Job drawing, mm, ordinate dimensions from the low corner. One solid piece. A direction names the side the tool comes from. Give positions to 0.01 mm unless a question says otherwise; leave off trailing zeros. Write each loop counter-clockwise with the first axis right and the second up, starting at its lowest first coordinate (ties: lowest second). Pieces come first, ordered by that corner, then holes. Notation, with made-up numbers: M 53.5,86 L 60.5,86 A37 ccw 60.5,124 Z; hole C 47.25,87.5 d8. An arc over 180 degrees is marked long. Answer as CSV lines item,"result". Start each with the question number.
Item 1: 3-axis set-ups, long thin cutter, end or side, ignore diameter. For the marked faces 5 and 6: which of +Z, -Z, +X, -X, +Y, -Y reach the whole face in a straight line?
Item 2: Wall check: L1, parallel to X at y = 33, z = 95.5 (3 decimals); L2, parallel to Z at x = 331, y = 35.5; L3, parallel to Z at x = 318, y = 17 (3 decimals). Give the ranges that are in metal, low to high. Write a range as from..to.
Item 3: Pin check, flat tips, straight feed: pin 1 (6 mm diameter, centred on x = 95.5, z = 20, fed in from -Y) (3 decimals); pin 2 (3 mm diameter, centred on x = 131.5, y = 14, fed in from -Z) (3 decimals). Stop position of each tip, or through.
Item 4: Band-saw the part on D-D, the plane y = 31. List the corners of the cut face in (x, z) (3 decimals), then the cut area to 3 significant figures.
Item 5: Band-saw the part on B-B, the plane z = 93. List the corners of the cut face in (x, y) (3 decimals).
Item 6: Band-saw the part on C-C, the plane z = 125. List the corners of the cut face in (x, y) (3 decimals).
Item 7: Band-saw the part on A-A, the plane x = 223. List the corners of the cut face in (y, z) (3 decimals), then the cut area to 3 significant figures.
Item 8: Two-plate mould, pull along X, no slides. Class the marked faces 1, 2, 3 and 4: +X half, -X half, draft (parallel to the pull), parting line (faces both ways), or undercut.
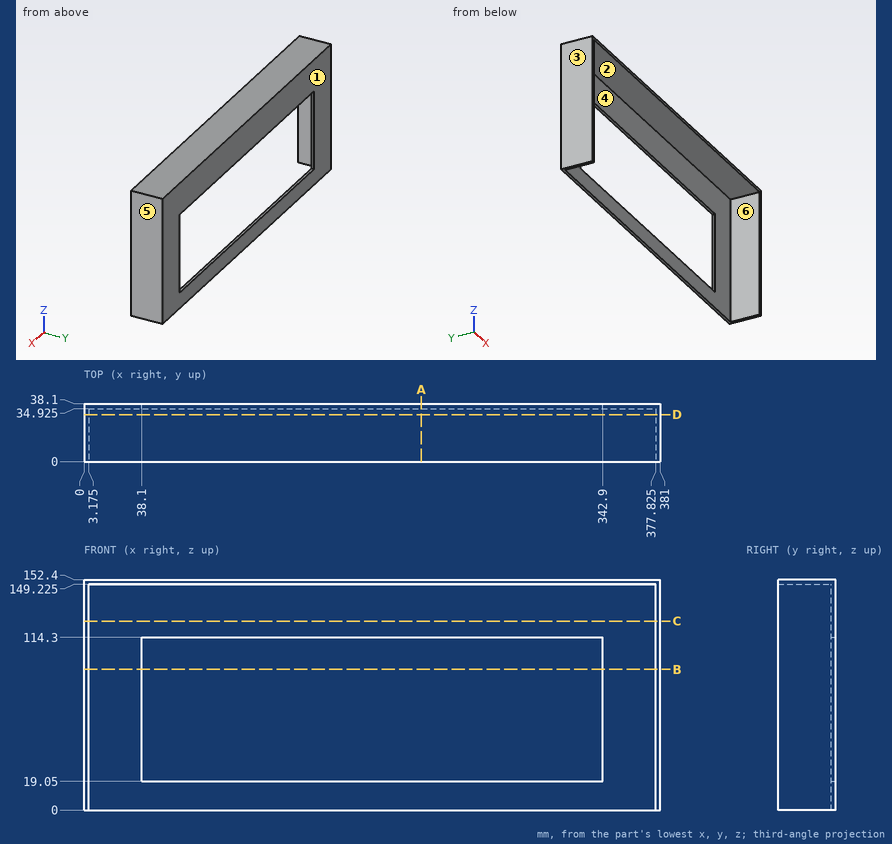
Output:
1,face 5,"+Z, -Z, +X, +Y, -Y"
1,face 6,"-Z, -Y"
2,L1,"0..3.175, 377.825..381"
2,L2,"0..19.05, 114.3..152.4"
2,L3,"149.225..152.4"
3,pin 1,"y = 34.925"
3,pin 2,"z = 149.225"
4,outline,"M 0,0 L 3.175,0 L 3.175,149.225 L 377.825,149.225 L 377.825,0 L 381,0 L 381,152.4 L 0,152.4 Z"
4,area,"2,160 mm²"
5,outline,"M 0,0 L 3.175,0 L 3.175,34.925 L 38.1,34.925 L 38.1,38.1 L 0,38.1 Z; M 342.9,34.925 L 377.825,34.925 L 377.825,0 L 381,0 L 381,38.1 L 342.9,38.1 Z"
6,outline,"M 0,0 L 3.175,0 L 3.175,34.925 L 377.825,34.925 L 377.825,0 L 381,0 L 381,38.1 L 0,38.1 Z"
7,outline,"M 0,149.225 L 34.925,149.225 L 34.925,114.3 L 38.1,114.3 L 38.1,152.4 L 0,152.4 Z; M 34.925,0 L 38.1,0 L 38.1,19.05 L 34.925,19.05 Z"
7,area,"292 mm²"
8,face 1,"draft"
8,face 2,"undercut"
8,face 3,"-X half"
8,face 4,"undercut"
